Part print with two shaded views. Sizes in mm from the minimum x, y, z corner. A direction names the side the tool comes from. Give positions to 0.01 mm unless a question says otherwise; leave off trailing zeros. Loops run counter-clockwise (first coordinate to the right, second up) from the corner with the lowest first, then second, coordinate; pieces in that order, holes last. Notation, with made-up numbers: M 12,56.5 L 53,56.5 A23 cw 53,66.5 Z; hole C 19,19.5 d8. An arc over 180 degrees is marked long. Answer in a Markdown table with one row per item.
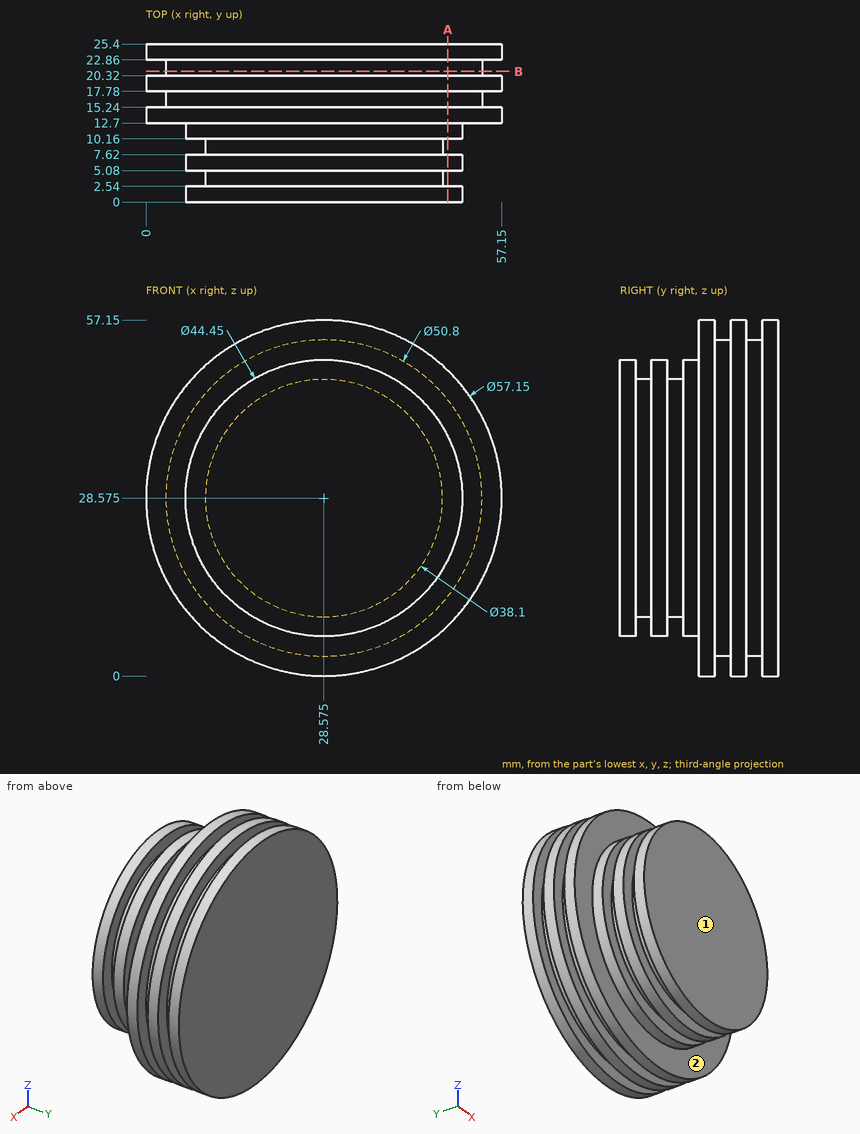
Q1. Probe probe 1 along Y at (x, z) = (55, 23.5); probe 2 along Y at (x, z) = (11, 17); probe 3 along Y at (x, z) = (37, 5). List the from-to ranges inside material, lowest first.
Reported:
| item | result |
|---|---|
| probe 1 | 12.7 to 15.24, 17.78 to 20.32, 22.86 to 25.4 |
| probe 2 | 0 to 2.54, 5.08 to 7.62, 10.16 to 25.4 |
| probe 3 | 12.7 to 25.4 |
Q2. Drop flat-ended pins along their axis: pin 1 (3 mm diameter, centred on x = 35.5, y = 11, fed in from -Z); pin 2 (10 mm diameter, centred on y = 12.5, z = 25, fed in from +X); pin 3 (4 mm diameter, centred on x = 11, y = 16.5, fed in from +Z). Give the stop position or say it passes through.
Reported:
| item | result |
|---|---|
| pin 1 | z = 7.02 |
| pin 2 | x = 57.15 |
| pin 3 | z = 52.24 |
Q3. Saw through at B-B (y = 21). Give the cut face in (x, z) (3 decimals).
Reported:
| item | result |
|---|---|
| outline | C 28.575,28.575 d50.8 |
Q4. Saw through at A-A (x = 48.5). Give the number of separate pieces and of enclosed holes in the cut face, and give its area (3 significant figures).
Reported:
| item | result |
|---|---|
| separate pieces | 3 |
| enclosed holes | 0 |
| area | 622 mm² |
Q5. 3-axis set-ups, long thin cutter, end or side, ignore diameter. For the marked faces 1 and 2: which of +Z, -Z, +X, -X, +Y, -Y reach the whole face in a straight line?
Reported:
| item | result |
|---|---|
| face 1 | +Z, -Z, +X, -X, -Y |
| face 2 | -Y |
